Read the model definition and answer for the solid it produces. Units are mm, in the model's axes. A direction names the side the tool comes from. Coordinates: 2 decimals unless noted, no trailing zeros. Order: outer loops, then holes, each group sorted by start corner. A loop starts at its lowest first (then second) coordinate and runs counter-clockwise, first axis right, second up. Notation, with made-up numbers: (48.25, -31.75) - (68.25, -31.75) arc R17 cw to (68.25, -21.75) - close; hole circle Ø4 at (5.5, 33.5). An arc over 180 degrees is marked (long way). Write item = value, one per line.
from build123d import *

# Parameters (mm, degrees)
EXTRUDE_1_DEPTH     = 25
SKETCH_2_W          = 10
SKETCH_2_H          = 25
EXTRUDE_2_DEPTH     = 5
FILLET_1_R          = 1
SKETCH_3_R          = 1.6
CUT_EXTRUDE_1_DEPTH = 20.5
FILLET_2_R          = 1


with BuildPart() as part:
    # Эскиз1 → Бобышка-Вытянуть1 (new body)
    with BuildSketch(Plane(origin=(0, 0, 0), x_dir=(1, 0, 0), z_dir=(0, 1, 0))):
        Polygon((0, 0), (43, 0), (43, 19.5), (38.25, 19.5), (38.25, 4.75), (4.75, 4.75), (4.75, 19.5), (0, 19.5), align=None)
    extrude(amount=EXTRUDE_1_DEPTH)

    # Эскиз2 → Бобышка-Вытянуть2 (add)
    with BuildSketch(Plane(origin=(0, 0, -19.5), x_dir=(-1, 0, 0), z_dir=(0, 0, -1))):
        with Locations((-48, 12.5)):
            Rectangle(SKETCH_2_W, SKETCH_2_H)
        with Locations((5, 12.5)):
            Rectangle(SKETCH_2_W, SKETCH_2_H)
    extrude(amount=-EXTRUDE_2_DEPTH)

    # Скругление1
    fillet_1_edges = [part.edges().sort_by_distance(p)[0] for p in [
        (4.75, 12.5, -4.75),
        (38.25, 12.5, -4.75),
    ]]
    fillet(fillet_1_edges, radius=FILLET_1_R)

    # Эскиз3 → Вырез-Вытянуть1 (cut, through all)
    with BuildSketch(Plane(origin=(0, 0, -19.5), x_dir=(-1, 0, 0), z_dir=(0, 0, -1))):
        with Locations((5, 20)):
            Circle(SKETCH_3_R)
        with Locations((5, 5)):
            Circle(SKETCH_3_R)
        with Locations((-48, 20)):
            Circle(SKETCH_3_R)
        with Locations((-48, 5)):
            Circle(SKETCH_3_R)
    extrude(amount=-CUT_EXTRUDE_1_DEPTH, mode=Mode.SUBTRACT)

    # Скругление2
    fillet_2_edges = [part.edges().sort_by_distance(p)[0] for p in [
        (0, 12.5, 0),
        (43, 12.5, 0),
    ]]
    fillet(fillet_2_edges, radius=FILLET_2_R)


solid = part.part
1) Determine the mould class of faces 5 (the face through (53, 12, -17)), 6 (the face through (46.52, 4.39, -17.04)), 7 (the face through (22, 25, -3)) for opening direction Y: pulls with the +Y half, pulls with the -Y half, needs draft (parallel to the pull), parting line crosses it, or undercut.
Returned:
face_5 = needs draft
face_6 = undercut
face_7 = pulls with the +Y half
2) The part is cut by section C-C (y = 20). Determine the outline of the cut face in (x, z).
Returned:
outline = (-10, -19.5) - (-6.6, -19.5) - (-6.6, -14.5) - (-10, -14.5) - close; (-3.4, -19.5) - (4.75, -19.5) - (4.75, -5.75) arc R1 cw to (5.75, -4.75) - (37.25, -4.75) arc R1 cw to (38.25, -5.75) - (38.25, -19.5) - (46.4, -19.5) - (46.4, -14.5) - (43, -14.5) - (43, -1) arc R1 ccw to (42, 0) - (1, 0) arc R1 ccw to (0, -1) - (0, -14.5) - (-3.4, -14.5) - close; (49.6, -19.5) - (53, -19.5) - (53, -14.5) - (49.6, -14.5) - close
3) Flat-ended cylindrical pins translate along their axes: pin 1 Ø4 at (y, z) = (10, -10.5) entering from +X; pin 2 Ø1.5 at (y, z) = (3.5, -4.5) entering from -X; pin 3 Ø1.9 at (x, y) = (-5, 5) entering from -Z; pin 4 Ø12.5 at (x, y) = (25, 10.5) entering from -Z. Find the tip coordinate at first contact, or state that the pin passes through.
Returned:
pin_1 = 43
pin_2 = 0
pin_3 = through
pin_4 = -4.75
4) The part is cut by section B-B (z = -15.25). Determine the outline of the cut face in (x, y), and give its area (3 significant figures).
Returned:
outline = (-10, 0) - (4.75, 0) - (4.75, 25) - (-10, 25) - close; (38.25, 0) - (53, 0) - (53, 25) - (38.25, 25) - close; hole circle Ø3.2 at (-5, 5); hole circle Ø3.2 at (-5, 20); hole circle Ø3.2 at (48, 5); hole circle Ø3.2 at (48, 20)
area = 705 mm^2
5) The part is cut by section A-A (z = -11.25). Determine the outline of the cut face in (x, y).
Returned:
outline = (0, 0) - (4.75, 0) - (4.75, 25) - (0, 25) - close; (38.25, 0) - (43, 0) - (43, 25) - (38.25, 25) - close
6) The part is cut by section D-D (x = 48). Determine the outline of the cut face in (y, z), and give its area (3 significant figures).
Returned:
outline = (0, -19.5) - (3.4, -19.5) - (3.4, -14.5) - (0, -14.5) - close; (6.6, -19.5) - (18.4, -19.5) - (18.4, -14.5) - (6.6, -14.5) - close; (21.6, -19.5) - (25, -19.5) - (25, -14.5) - (21.6, -14.5) - close
area = 93.0 mm^2
7) For faces 1 (the face through (0, 12, -8)), 2 (the face through (47.14, 21.35, -17.04)), 3 (the face through (22, 12, -4.75)), 4 (the face through (48, 13, -14.5)), determine the directions among +Z, -Z, +X, -X, +Y, -Y from which every point of the face is accessible in a straight line to the end or side of a thin tool.
Returned:
face_1 = +Z, -X, +Y, -Y
face_2 = +Z, -Z
face_3 = -Z, +Y, -Y
face_4 = +Z, +X, +Y, -Y
8) Straight lines are drawn through the part: line 1 along Y through (x, z) = (-5, -16.7); line 2 along X through (y, z) = (8, -11.5); line 3 along Z through (x, y) = (20.5, 8.25). For each, find the intervals that lie inside material, in ascending order. Write a range as from..to.
Returned:
line_1 = 0..3.4, 6.6..18.4, 21.6..25
line_2 = 0..4.75, 38.25..43
line_3 = -4.75..0
